```python
from build123d import *

# Parameters (mm, degrees)
SKETCH3_W           = 70
SKETCH3_H           = 37
BOSS_EXTRUDE1_DEPTH = 6
FILLET1_R           = 2
SKETCH4_R           = 2.5
CUT_EXTRUDE1_DEPTH  = 5
SKETCH4_3_R         = 2.5
CUT_EXTRUDE2_DEPTH  = 5
SKETCH4_5_R         = 2.5
CUT_EXTRUDE3_DEPTH  = 5
CHAMFER1_SIZE       = 1


with BuildPart() as part:
    # Sketch3 → Boss-Extrude1 (new body)
    with BuildSketch(Plane(origin=(0, 0, 0), x_dir=(1, 0, 0), z_dir=(0, 1, 0))):
        Rectangle(SKETCH3_W, SKETCH3_H)
    extrude(amount=BOSS_EXTRUDE1_DEPTH)

    # Fillet1
    fillet1_edges = [part.edges().sort_by_distance(p)[0] for p in [
        (-35, 3, 18.5),
        (35, 3, 18.5),
        (35, 3, -18.5),
        (-35, 3, -18.5),
    ]]
    fillet(fillet1_edges, radius=FILLET1_R)

    # Sketch4 → Cut-Extrude1 (cut)
    with BuildSketch(Plane(origin=(0, 6, 0), x_dir=(1, 0, 0), z_dir=(0, 1, 0))):
        with Locations(Location((28, -5.39, 0), (0, 0, 270))):
            Circle(SKETCH4_R)
    extrude(amount=-CUT_EXTRUDE1_DEPTH, mode=Mode.SUBTRACT)

    # Sketch4_3 → Cut-Extrude2 (cut)
    with BuildSketch(Plane(origin=(0, 6, 0), x_dir=(1, 0, 0), z_dir=(0, 1, 0))):
        with Locations(Location((14.24, 5.39, 0), (0, 0, 270))):
            Circle(SKETCH4_3_R)
    extrude(amount=-CUT_EXTRUDE2_DEPTH, mode=Mode.SUBTRACT)

    # Sketch4_5 → Cut-Extrude3 (cut)
    with BuildSketch(Plane(origin=(0, 6, 0), x_dir=(1, 0, 0), z_dir=(0, 1, 0))):
        with Locations(Location((-28, 0, 0), (0, 0, 270))):
            Circle(SKETCH4_5_R)
    extrude(amount=-CUT_EXTRUDE3_DEPTH, mode=Mode.SUBTRACT)

    # Chamfer1
    chamfer1_edges = [part.edges().sort_by_distance(p)[0] for p in [
        (28, 6, 2.89),
        (14.24, 6, -7.89),
        (-28, 6, -2.5),
    ]]
    chamfer(chamfer1_edges, length=CHAMFER1_SIZE)


solid = part.part
```
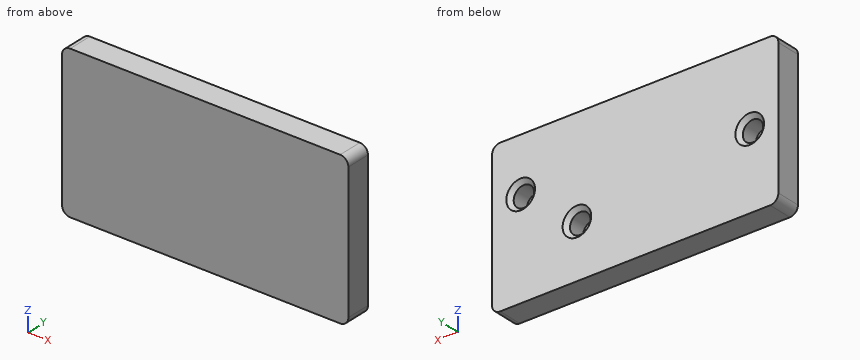
Geometry check sheet. Reference: the model listing, model coordinates, mm. Round coordinates to 2 decimals unless told otherwise and drop trailing zeros. Order: outer loops, then holes, each group sorted by start corner. A loop starts at its lowest first (then second) coordinate and runs counter-clockwise, first axis right, second up. Notation, with made-up numbers: (15.25, 30) -> (61.25, 30) arc R31 ccw to (61.25, 67) -> close; hole circle Ø8 at (85, 79). An arc over 180 degrees is marked (long way). Return JSON: item names as keys, results as strings. Group by question number.
Q1. Section check B-B, the plane y = 2.15. Record the boundary of the cut face in (x, z).
Q2. Section check C-C, the plane z = 0. Record the boundary of the cut face in (x, y), plus the area to 3 significant figures.
Q3. Material ranges on probe 1 along X at (y, z) = (2.25, 0); probe 2 along X at (y, z) = (3.3, 0.5); probe 3 along Z at (x, y) = (30, 2.9), recorded low to high. Write a range as from..to.
Q4. Section check A-A, the plane x = -28. Record the boundary of the cut face in (y, z).
Q5. Gauge pin test, flat ends, axial feed: pin 1 (5 mm diameter, centred on x = 27.5, z = 12, fed in from -Y); pin 2 (1.5 mm diameter, centred on x = -28, z = 1, fed in from +Y). Record the tip position at first contact, or that the pin passes through.
Numbers:
{
 "1": {"outline": "(-35, -16.5) arc R2 ccw to (-33, -18.5) -> (33, -18.5) arc R2 ccw to (35, -16.5) -> (35, 16.5) arc R2 ccw to (33, 18.5) -> (-33, 18.5) arc R2 ccw to (-35, 16.5) -> close; hole circle Ø5 at (-28, 0); hole circle Ø5 at (14.24, -5.39); hole circle Ø5 at (28, 5.39)"},
 "2": {"outline": "(-35, 0) -> (35, 0) -> (35, 6) -> (-24.5, 6) -> (-25.5, 5) -> (-25.5, 1) -> (-30.5, 1) -> (-30.5, 5) -> (-31.5, 6) -> (-35, 6) -> close", "area": "394 mm^2"},
 "3": {"probe 1": "-35..-30.5, -25.5..35", "probe 2": "-35..-30.45, -25.55..35", "probe 3": "-18.5..3.89, 6.89..18.5"},
 "4": {"outline": "(0, -18.5) -> (6, -18.5) -> (6, -3.5) -> (5, -2.5) -> (1, -2.5) -> (1, 2.5) -> (5, 2.5) -> (6, 3.5) -> (6, 18.5) -> (0, 18.5) -> close"},
 "5": {"pin 1": "y = 0", "pin 2": "y = 1"}
}
